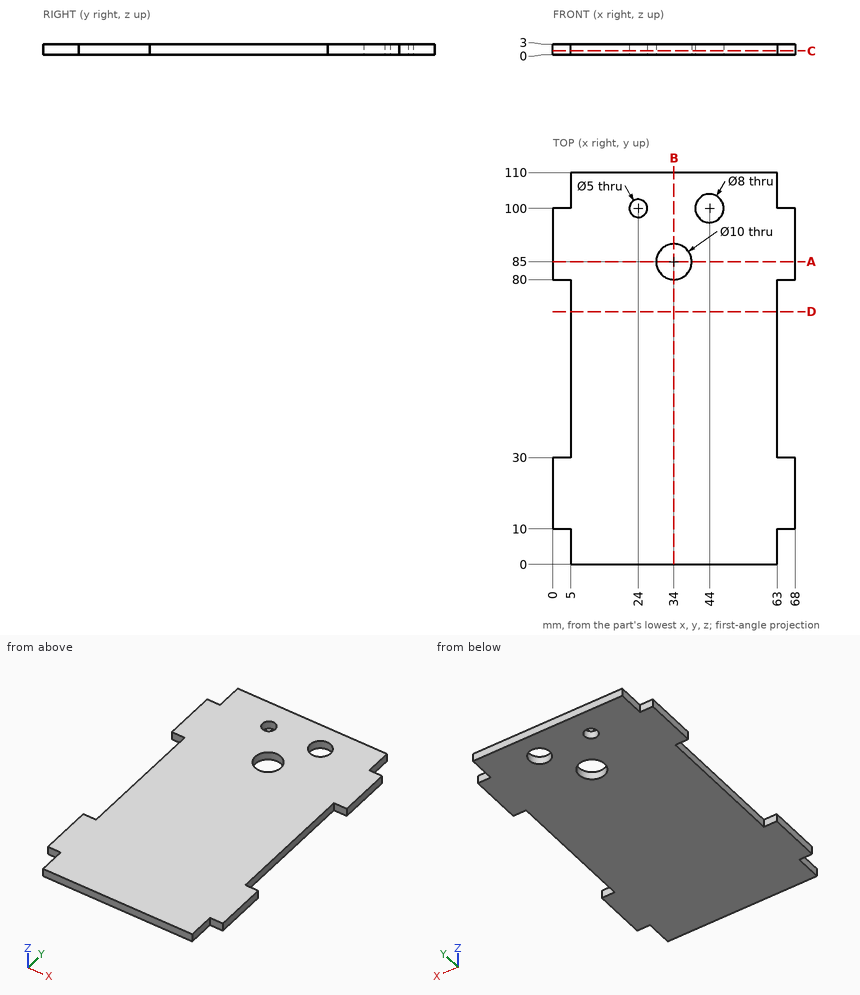
The figure shows three views and two pictorial views of one solid part (mm, origin at its lowest corner). Answer the questions. Coordinates: 2 decimals unless noted, no trailing zeros. Loops run counter-clockwise (first coordinate to the right, second up) from the corner with the lowest first, then second, coordinate; pieces in that order, holes last. Notation, with made-up numbers: (35, 47.5) - (82, 47.5) arc R20 ccw to (82, 63.5) - close; hole circle Ø6 at (-3.75, 5). An arc over 180 degrees is marked (long way). Answer in a Markdown table with one row per item.
Q1. Find section A-A on y = 85. Write down the section's boundary in (x, z), plus the area to 3 significant figures.
Here are the results:
| item | result |
|---|---|
| outline | (0, 0) - (29, 0) - (29, 3) - (0, 3) - close; (39, 0) - (68, 0) - (68, 3) - (39, 3) - close |
| area | 174 mm^2 |
Q2. Find section C-C on z = 1.05. Write down the section's boundary in (x, y).
Here are the results:
| item | result |
|---|---|
| outline | (0, 10) - (5, 10) - (5, 0) - (63, 0) - (63, 10) - (68, 10) - (68, 30) - (63, 30) - (63, 80) - (68, 80) - (68, 100) - (63, 100) - (63, 110) - (5, 110) - (5, 100) - (0, 100) - (0, 80) - (5, 80) - (5, 30) - (0, 30) - close; hole circle Ø5 at (24, 100); hole circle Ø10 at (34, 85); hole circle Ø8 at (44, 100) |
Q3. Straight lines are drawn through the part: line 1 along Y through (x, z) = (24, 2.35); line 2 along Y through (x, z) = (44, 2.4); line 3 along X through (y, z) = (43, 0.35). For each, find the intervals that lie inside material, in ascending order. Write a range as [from, to].
Here are the results:
| item | result |
|---|---|
| line 1 | y = [0, 97.5], [102.5, 110] |
| line 2 | y = [0, 96], [104, 110] |
| line 3 | x = [5, 63] |
Q4. Given P1, Ø1.5, axis at y = 103.5, z = 1.5, coming from the -X side; P2, Ø1.5, axis at x = 3.5, z = 1, coming from the -Y side; P3, Ø0.9, axis at y = 104, z = 1, coming from the +X side, each flat-ended and moving along its own axis, determine where each tip first touches the part or whether it passes through.
Here are the results:
| item | result |
|---|---|
| P1 | stops at x = 5 |
| P2 | stops at y = 10 |
| P3 | stops at x = 63 |
Q5. Find section D-D on y = 71. Write down the section's boundary in (x, z).
Here are the results:
| item | result |
|---|---|
| outline | (5, 0) - (63, 0) - (63, 3) - (5, 3) - close |
Q6. Find section B-B on x = 34. Write down the section's boundary in (y, z).
Here are the results:
| item | result |
|---|---|
| outline | (0, 0) - (80, 0) - (80, 3) - (0, 3) - close; (90, 0) - (110, 0) - (110, 3) - (90, 3) - close |
